Verification items for the finished model (mm, model axes). A direction names the side the tool comes from. Give positions to 0.01 mm unless a question says otherwise; leave off trailing zeros. Write each loop counter-clockwise with the first axis right and the second up, starting at its lowest first coordinate (ties: lowest second). Pieces come first, ordered by that corner, then holes. Notation, with made-up numbers: (-13.75, -16) -> (20.25, -16) arc R32 cw to (20.25, 10) -> close; hole circle Ø6 at (-26, 63.25). An arc over 180 degrees is marked (long way). Write item = value, one per line.
from build123d import *

# Parameters (mm, degrees)
SALIENTE_EXTRUIR1_DEPTH    = 22.5
CROQUIS2_W                 = 7
CROQUIS2_H                 = 38
SALIENTE_EXTRUIR2_DEPTH    = 65
CORTAR_EXTRUIR1_DEPTH      = 81.854808144
CORTAR_EXTRUIR1_DEPTH_BACK = 81.854808144
CROQUIS3_R                 = 1.5


with BuildPart() as part:
    # Croquis1 → Saliente-Extruir1 (new body)
    with BuildSketch(Plane.XY):
        Polygon((-15, 21.5), (-21.5, 15), (-21.5, -15), (-15, -21.5), (15, -21.5), (21.5, -15), (21.5, 15), (15, 21.5), (2, 21.5), (2, 34.5), (5.5, 34.5), (12.25, 26.5), (19, 26.5), (26.5, 19), (26.5, -19), (19, -26.5), (-19, -26.5), (-26.5, -19), (-26.5, 19), (-19, 26.5), (-12.25, 26.5), (-5.5, 34.5), (-2, 34.5), (-2, 21.5), align=None)
    extrude(amount=SALIENTE_EXTRUIR1_DEPTH)

    # Croquis2 → Saliente-Extruir2 (add)
    with BuildSketch(Plane.XY):
        with Locations((-30, 0)):
            Rectangle(CROQUIS2_W, CROQUIS2_H)
    extrude(amount=SALIENTE_EXTRUIR2_DEPTH)

    # Croquis3 → Cortar-Extruir1 (cut, two sides: drawn at the far end of the back side and taken through both)
    with BuildSketch(Plane(origin=(0, 0, 0), x_dir=(0, 0, -1), z_dir=(1, 0, 0)).offset(-CORTAR_EXTRUIR1_DEPTH_BACK)):
        with Locations(Location((-11.25, 30.5, 0), (0, 0, 90))):
            Circle(CROQUIS3_R)
        with Locations((-53, 12)):
            Circle(CROQUIS3_R)
        with Locations((-34.2, 12)):
            Circle(CROQUIS3_R)
        with Locations((-34.2, -12)):
            Circle(CROQUIS3_R)
        with Locations((-53, -12)):
            Circle(CROQUIS3_R)
    extrude(amount=CORTAR_EXTRUIR1_DEPTH + CORTAR_EXTRUIR1_DEPTH_BACK, mode=Mode.SUBTRACT)


solid = part.part
Item 1: Sectioned sample at A-A on y = -17. Record the cut outline in (x, z), then the cut area to 3 significant figures.
Response values:
outline = (-33.5, 0) -> (-19.5, 0) -> (-19.5, 22.5) -> (-26.5, 22.5) -> (-26.5, 65) -> (-33.5, 65) -> close; (19.5, 0) -> (26.5, 0) -> (26.5, 22.5) -> (19.5, 22.5) -> close
area = 770 mm^2
Item 2: Sectioned sample at B-B on x = -16.5. Record the cut outline in (y, z), then the cut area to 4 significant figures.
Response values:
outline = (-26.5, 0) -> (-20, 0) -> (-20, 22.5) -> (-26.5, 22.5) -> close; (20, 0) -> (26.5, 0) -> (26.5, 22.5) -> (20, 22.5) -> close
area = 292.5 mm^2
Item 3: Mould release check, pull along Y, two halves, no side actions. Record for faces 1 (the flat face through (-16, 26.5, 11)), 2 (the flat face through (2, 28, 11)), 3 (the cylindrical face through (-30, 11.1, 54.2)): +Y half, -Y half, draft (parallel to the pull), parting line (faces both ways), or undercut.
Response values:
face_1 = +Y half
face_2 = draft
face_3 = undercut
Item 4: Sectioned sample at D-D on y = 23. Record the cut outline in (x, z).
Response values:
outline = (-22.5, 0) -> (-2, 0) -> (-2, 22.5) -> (-22.5, 22.5) -> close; (2, 0) -> (22.5, 0) -> (22.5, 22.5) -> (2, 22.5) -> close
Item 5: Go/stop test with flat-tipped pins: P1, Ø6.5, axis at y = 29.5, z = 14.5, coming from the +X side; P2, Ø2, axis at y = 1, z = 37.5, coming from the +X side; P3, Ø5, axis at y = 26, z = 24, coming from the +X side. Record where each tip stops, or that it passes through.
Response values:
P1 = 19.25
P2 = -26.5
P3 = 21.5
Item 6: Material ranges on line 1 (Z direction, x = -29.5, y = 12); line 2 (Y direction, x = -28, z = 53); line 3 (Y direction, x = 7, z = 11.25), recorded low to high.
Response values:
line_1 = 0 to 32.7, 35.7 to 51.5, 54.5 to 65
line_2 = -19 to -13.5, -10.5 to 10.5, 13.5 to 19
line_3 = -26.5 to -21.5, 21.5 to 29, 32 to 32.72
Item 7: Sectioned sample at C-C on z = 34.2. Record the cut outline in (x, y).
Response values:
outline = (-33.5, -19) -> (-26.5, -19) -> (-26.5, -13.5) -> (-33.5, -13.5) -> close; (-33.5, -10.5) -> (-26.5, -10.5) -> (-26.5, 10.5) -> (-33.5, 10.5) -> close; (-33.5, 13.5) -> (-26.5, 13.5) -> (-26.5, 19) -> (-33.5, 19) -> close
Item 8: Set-up check for faces 4 (the cylindrical face through (-30.05, -11.55, 32.77)), 5 (the flat face through (-30, -19, 32)), 6 (the flat face through (18.2, -18.3, 11.1)), 7 (the flat face through (-30, 19, 32)): record each of +Z, -Z, +X, -X, +Y, -Y from which the full face is reachable in a straight line by a thin tool's end or side.
Response values:
face_4 = +X, -X
face_5 = +Z, -Z, -X, -Y
face_6 = +Z, -Z
face_7 = +Z, -Z, -X, +Y
